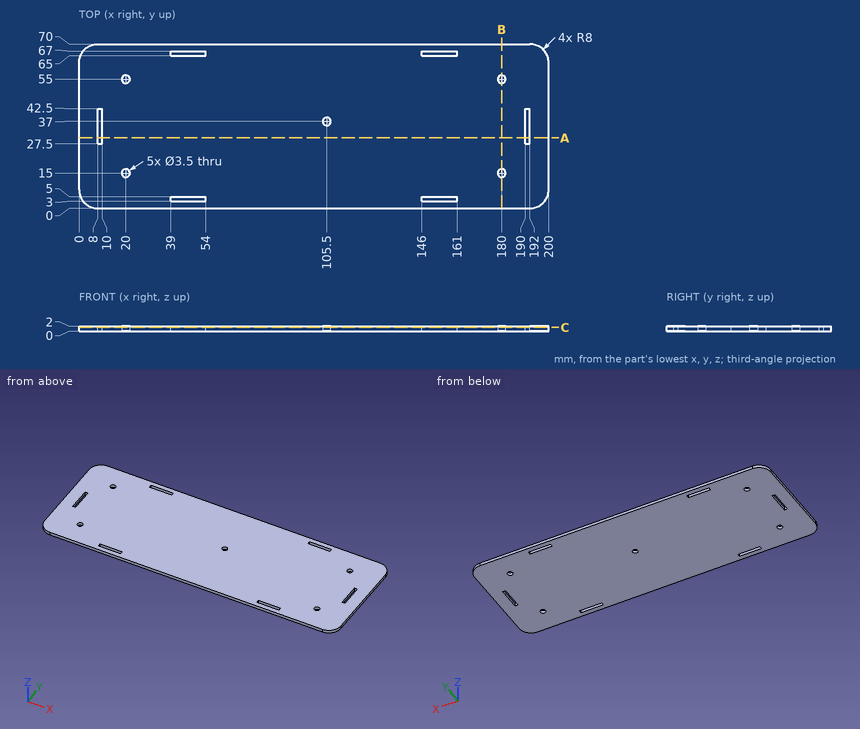
Drawing for the job (mm, zero at the part's lowest x, y, z). Round coordinates to 2 decimals unless told otherwise and drop trailing zeros. Loops run counter-clockwise (first coordinate to the right, second up) from the corner with the lowest first, then second, coordinate; pieces in that order, holes last. Notation, with made-up numbers: M 34.5,14 L 57.5,14 A13 ccw 57.5,35 Z; hole C 24,11.5 d9. An arc over 180 degrees is marked long. Use a Markdown table: item, result. Add a question column.
(1) Cut at B-B (x = 180). Give the cut face in (y, z).
(2) Cut at C-C (z = 1.55). State how many separate pieces and enclosed holes the cut face has, and give its area (3 significant figures).
(3) Cut at A-A (y = 30). Give the cut face in (x, z), and give its area (3 significant figures).
(4) Drill centre lines: line 1 (X direction, y = 30.5, z = 1.85); line 2 (Y direction, x = 180, z = 1.55); line 3 (Y direction, x = 42.5, z = 0.5). Where is each one in solid material? Low to high.
(5) Flat gauge pins, fed straight in: pin 1 (1 mm diameter, centred on x = 59.5, y = 24, fed in from -Z); pin 2 (1 mm diameter, centred on y = 65.5, z = 1, fed in from +X); pin 3 (0.6 mm diameter, centred on y = 66, z = 1.5, fed in from +X); pin 4 (0.6 mm diameter, centred on y = 66.5, z = 1, fed in from -X). Where does each tip first touch, or does it go through?
Geometry says:
| question | item | result |
|---|---|---|
| 1 | outline | M 0,0 L 13.25,0 L 13.25,2 L 0,2 Z; M 16.75,0 L 53.25,0 L 53.25,2 L 16.75,2 Z; M 56.75,0 L 70,0 L 70,2 L 56.75,2 Z |
| 2 | separate pieces | 1 |
| 2 | enclosed holes | 11 |
| 2 | area | 13,700 mm² |
| 3 | outline | M 0,0 L 8,0 L 8,2 L 0,2 Z; M 10,0 L 190,0 L 190,2 L 10,2 Z; M 192,0 L 200,0 L 200,2 L 192,2 Z |
| 3 | area | 392 mm² |
| 4 | line 1 | x = 0 to 8, 10 to 190, 192 to 200 |
| 4 | line 2 | y = 0 to 13.25, 16.75 to 53.25, 56.75 to 70 |
| 4 | line 3 | y = 0 to 3, 5 to 65, 67 to 70 |
| 5 | pin 1 | stops at z = 0 |
| 5 | pin 2 | stops at x = 199.42 |
| 5 | pin 3 | stops at x = 199.09 |
| 5 | pin 4 | stops at x = 1.19 |
